Read the model definition and answer for the solid it produces. Units are mm, in the model's axes. A direction names the side the tool comes from. Round coordinates to 2 decimals unless told otherwise and drop trailing zeros. Loops run counter-clockwise (first coordinate to the right, second up) from the corner with the lowest first, then second, coordinate; pieces in that order, holes last. Notation, with made-up numbers: M -37.5,72 L -5.5,72 A23 ccw -5.5,110 Z; hole C 75,39 d4. An arc over 180 degrees is marked long. Answer as CSV lines item,"result".
```python
from build123d import *

# Parameters (mm, degrees)
SKETCH1_R           = 120.65
SKETCH1_R_2         = 7.5
SKETCH1_R_3         = 4
BOSS_EXTRUDE1_DEPTH = 2
SKETCH2_R           = 11.5
SKETCH2_R_2         = 7.5
BOSS_EXTRUDE2_DEPTH = 60
BOSS_EXTRUDE3_DEPTH = 2
CHAMFER1_SIZE       = 3
CHAMFER8_SIZE       = 2


with BuildPart() as part:
    # Sketch1 → Boss-Extrude1 (new body)
    with BuildSketch(Plane(origin=(0, 0, 0), x_dir=(1, 0, 0), z_dir=(0, 1, 0))):
        with Locations(Location((0, 0, 0), (0, 0, 270))):
            Circle(SKETCH1_R)
        with Locations(Location((0, 0, 0), (0, 0, 270))):
            Circle(SKETCH1_R_2, mode=Mode.SUBTRACT)
        with Locations(Location((-85, 0, 0), (0, 0, 270))):
            Circle(SKETCH1_R_3, mode=Mode.SUBTRACT)
        with Locations(Location((-42.5, 73.612159322, 0), (0, 0, 270))):
            Circle(SKETCH1_R_3, mode=Mode.SUBTRACT)
        with Locations(Location((42.5, 73.612159322, 0), (0, 0, 270))):
            Circle(SKETCH1_R_3, mode=Mode.SUBTRACT)
        with Locations(Location((85, 0, 0), (0, 0, 270))):
            Circle(SKETCH1_R_3, mode=Mode.SUBTRACT)
        with Locations(Location((42.5, -73.612159322, 0), (0, 0, 270))):
            Circle(SKETCH1_R_3, mode=Mode.SUBTRACT)
        with Locations(Location((-42.5, -73.612159322, 0), (0, 0, 270))):
            Circle(SKETCH1_R_3, mode=Mode.SUBTRACT)
        with Locations(Location((-110, 0, 0), (0, 0, 270))):
            Circle(SKETCH1_R_3, mode=Mode.SUBTRACT)
        with Locations(Location((-55, 95.262794416, 0), (0, 0, 270))):
            Circle(SKETCH1_R_3, mode=Mode.SUBTRACT)
        with Locations(Location((55, 95.262794416, 0), (0, 0, 270))):
            Circle(SKETCH1_R_3, mode=Mode.SUBTRACT)
        with Locations(Location((110, 0, 0), (0, 0, 270))):
            Circle(SKETCH1_R_3, mode=Mode.SUBTRACT)
        with Locations(Location((55, -95.262794416, 0), (0, 0, 270))):
            Circle(SKETCH1_R_3, mode=Mode.SUBTRACT)
        with Locations(Location((-55, -95.262794416, 0), (0, 0, 270))):
            Circle(SKETCH1_R_3, mode=Mode.SUBTRACT)
        with Locations(Location((-11.320321377, 99.357185568, 0), (0, 0, 270))):
            Circle(SKETCH1_R_3, mode=Mode.SUBTRACT)
        with Locations(Location((11.320321377, 99.357185568, 0), (0, 0, 270))):
            Circle(SKETCH1_R_3, mode=Mode.SUBTRACT)
        with Locations(Location((91.706007439, 39.874906893, 0), (0, 0, 270))):
            Circle(SKETCH1_R_3, mode=Mode.SUBTRACT)
        with Locations(Location((80.385686062, 59.482278675, 0), (0, 0, 270))):
            Circle(SKETCH1_R_3, mode=Mode.SUBTRACT)
        with Locations(Location((80.385686062, -59.482278675, 0), (0, 0, 270))):
            Circle(SKETCH1_R_3, mode=Mode.SUBTRACT)
        with Locations(Location((91.706007439, -39.874906893, 0), (0, 0, 270))):
            Circle(SKETCH1_R_3, mode=Mode.SUBTRACT)
        with Locations(Location((-11.320321377, -99.357185568, 0), (0, 0, 270))):
            Circle(SKETCH1_R_3, mode=Mode.SUBTRACT)
        with Locations(Location((11.320321377, -99.357185568, 0), (0, 0, 270))):
            Circle(SKETCH1_R_3, mode=Mode.SUBTRACT)
        with Locations(Location((-91.706007439, -39.874906893, 0), (0, 0, 270))):
            Circle(SKETCH1_R_3, mode=Mode.SUBTRACT)
        with Locations(Location((-80.385686062, -59.482278675, 0), (0, 0, 270))):
            Circle(SKETCH1_R_3, mode=Mode.SUBTRACT)
        with Locations(Location((-80.385686062, 59.482278675, 0), (0, 0, 270))):
            Circle(SKETCH1_R_3, mode=Mode.SUBTRACT)
        with Locations(Location((-91.706007439, 39.874906893, 0), (0, 0, 270))):
            Circle(SKETCH1_R_3, mode=Mode.SUBTRACT)
    extrude(amount=BOSS_EXTRUDE1_DEPTH)

    # Sketch2 → Boss-Extrude2 (add)
    with BuildSketch(Plane(origin=(0, 2, 0), x_dir=(1, 0, 0), z_dir=(0, 1, 0))):
        with Locations(Location((0, 0, 0), (0, 0, 270))):
            Circle(SKETCH2_R)
        with Locations(Location((0, 0, 0), (0, 0, 270))):
            Circle(SKETCH2_R_2, mode=Mode.SUBTRACT)
    extrude(amount=BOSS_EXTRUDE2_DEPTH)

    # Sketch3 → Revolve1 (revolve)
    with BuildSketch(Plane.XY, mode=Mode.PRIVATE) as revolve1_sk:
        with BuildLine():
            Line((0, 0), (15, 0))
            ThreePointArc((15, 0), (14.880445444, -1.890064387), (14.523687548, -3.75))
            ThreePointArc((14.523687548, -3.75), (12.744320544, -6.452847075), (9.682458366, -7.5))
            Line((9.682458366, -7.5), (0, -7.5))
            Line((0, -7.5), (0, 0))
        make_face()
    revolve(revolve1_sk.sketch.rotate(Axis((0, 0, 0), (0, -1, 0)), 90), axis=Axis((0, 0, 0), (0, -1, 0)))

    # Sketch4 → Boss-Extrude3 (add)
    with BuildSketch(Plane.XZ):
        with BuildLine():
            Line((-19, 90), (19, 90))
            Line((19, 90), (19, 105))
            Line((19, 105), (0.479917223, 168.358177922))
            ThreePointArc((0.479917223, 168.358177922), (0, 168.717894426), (-0.479917223, 168.358177922))
            Line((-0.479917223, 168.358177922), (-19, 105))
            Line((-19, 105), (-19, 90))
        make_face()
        with BuildLine():
            Line((81.432667397, -68.954482672), (145.562500404, -84.594709468))
            ThreePointArc((145.562500404, -84.594709468), (146.113982646, -84.358947213), (146.042417627, -83.763468454))
            Line((146.042417627, -83.763468454), (100.432667397, -36.045517328))
            Line((100.432667397, -36.045517328), (87.442286341, -28.545517328))
            Line((87.442286341, -28.545517328), (68.442286341, -61.454482672))
            Line((68.442286341, -61.454482672), (81.432667397, -68.954482672))
        make_face()
        with BuildLine():
            Line((-100.432667397, -36.045517328), (-146.042417627, -83.763468454))
            ThreePointArc((-146.042417627, -83.763468454), (-146.113982646, -84.358947213), (-145.562500404, -84.594709468))
            Line((-145.562500404, -84.594709468), (-81.432667397, -68.954482672))
            Line((-81.432667397, -68.954482672), (-68.442286341, -61.454482672))
            Line((-68.442286341, -61.454482672), (-87.442286341, -28.545517328))
            Line((-87.442286341, -28.545517328), (-100.432667397, -36.045517328))
        make_face()
    extrude(amount=BOSS_EXTRUDE3_DEPTH)

    # Chamfer1
    chamfer1_edges = [part.edges().sort_by_distance(p)[0] for p in [
        (0, 2, -11.5),
    ]]
    chamfer(chamfer1_edges, length=CHAMFER1_SIZE)

    # Chamfer8
    # the kernel refuses this chamfer: 2 mm, written as the material it takes off along each edge
    with BuildSketch(Plane(origin=(-94.391126841, -2, -29.724721105), x_dir=(0, 1, 0), z_dir=(-0.690957517475874, 0, -0.7228953652110223)), Plane(origin=(-150.55940651, -2, -85.813373872), x_dir=(0, 1, 0), z_dir=(0.9715245092887052, 0, 0.2369390804644533)), Plane(origin=(0.963141497, -2, 173.294957752), x_dir=(0, 1, 0), z_dir=(-0.2805669918128247, 0, -0.9598344456754521)), Plane(origin=(21.453199823, -2, 96.607474288), x_dir=(0, 1, 0), z_dir=(-0.2805669918128244, 0, 0.9598344456754522)), Plane(origin=(149.596265013, -2, -87.48158388), x_dir=(0, 1, 0), z_dir=(-0.6909575174758892, 0, 0.7228953652110078)), Plane(origin=(72.937927017, -2, -66.882753184), x_dir=(0, 1, 0), z_dir=(0.9715245092887104, 0, -0.23693908046443202))) as chamfer8_piece_1:
        Polygon((CHAMFER8_SIZE, 0), (0, CHAMFER8_SIZE), (0, 0), align=None)
    extrude(amount=79.896573633, mode=Mode.SUBTRACT)
    with BuildSketch(Plane(origin=(145.680969944, -2, -84.108947213), x_dir=(-0.2369390804643702, 0, -0.9715245092887255), z_dir=(-0.9715245092887255, 0, 0.2369390804643702))) as chamfer8_piece_2_section:
        Polygon((0.5, -CHAMFER8_SIZE), (0, -1.5), (0, 0), (0.5, 0), align=None)
    chamfer8_piece_2 = revolve(axis=Axis((145.680969944, -2, -84.108947213), (0, -1, 0)), revolution_arc=147.411905087, mode=Mode.PRIVATE)
    chamfer8_piece_2 = split(chamfer8_piece_2, bisect_by=Plane(origin=(145.858674254, -1.25, -83.380303831), z_dir=(-0.16754123052450473, -0.7071067811865483, -0.6869715686069793)), keep=Keep.TOP, mode=Mode.PRIVATE)
    add(chamfer8_piece_2, mode=Mode.SUBTRACT)
    with BuildSketch(Plane(origin=(145.680969944, -2, -84.108947213), x_dir=(-0.2369390804643702, 0, -0.9715245092887255), z_dir=(-0.9715245092887255, 0, 0.2369390804643702))) as chamfer8_piece_3_section:
        Polygon((0.5, -CHAMFER8_SIZE), (0, -1.5), (0, 0), (0.5, 0), align=None)
    chamfer8_piece_3 = revolve(axis=Axis((145.680969944, -2, -84.108947213), (0, -1, 0)), revolution_arc=147.411905087, mode=Mode.PRIVATE)
    chamfer8_piece_3 = split(chamfer8_piece_3, bisect_by=Plane(origin=(145.13879842, -1.25, -84.627165351), z_dir=(0.5111642148290308, -0.7071067811865457, 0.4885807461190251)), keep=Keep.TOP, mode=Mode.PRIVATE)
    add(chamfer8_piece_3, mode=Mode.SUBTRACT)
    with BuildSketch(Plane(origin=(0, -2, 168.217894426), x_dir=(0.9598344456754415, 0, 0.2805669918128611), z_dir=(0.2805669918128611, 0, -0.9598344456754415))) as chamfer8_piece_4_section:
        Polygon((0.5, -CHAMFER8_SIZE), (0, -1.5), (0, 0), (0.5, 0), align=None)
    chamfer8_piece_4 = revolve(axis=Axis((0, -2, 168.217894426), (0, -1, 0)), revolution_arc=147.411905087, mode=Mode.PRIVATE)
    chamfer8_piece_4 = split(chamfer8_piece_4, bisect_by=Plane(origin=(-0.719875834, -1.25, 168.007469182), z_dir=(0.678705445353544, -0.7071067811865469, 0.19839082248795895)), keep=Keep.TOP, mode=Mode.PRIVATE)
    add(chamfer8_piece_4, mode=Mode.SUBTRACT)
    with BuildSketch(Plane(origin=(0, -2, 168.217894426), x_dir=(0.9598344456754415, 0, 0.2805669918128611), z_dir=(0.2805669918128611, 0, -0.9598344456754415))) as chamfer8_piece_5_section:
        Polygon((0.5, -CHAMFER8_SIZE), (0, -1.5), (0, 0), (0.5, 0), align=None)
    chamfer8_piece_5 = revolve(axis=Axis((0, -2, 168.217894426), (0, -1, 0)), revolution_arc=147.411905087, mode=Mode.PRIVATE)
    chamfer8_piece_5 = split(chamfer8_piece_5, bisect_by=Plane(origin=(0.719875834, -1.25, 168.007469182), z_dir=(-0.6787054453535436, -0.707106781186547, 0.19839082248795903)), keep=Keep.TOP, mode=Mode.PRIVATE)
    add(chamfer8_piece_5, mode=Mode.SUBTRACT)
    with BuildSketch(Plane(origin=(-145.680969944, -2, -84.108947213), x_dir=(-0.7228953652110097, 0, 0.6909575174758872), z_dir=(0.6909575174758872, 0, 0.7228953652110097))) as chamfer8_piece_6_section:
        Polygon((0.5, -CHAMFER8_SIZE), (0, -1.5), (0, 0), (0.5, 0), align=None)
    chamfer8_piece_6 = revolve(axis=Axis((-145.680969944, -2, -84.108947213), (0, -1, 0)), revolution_arc=147.411905087, mode=Mode.PRIVATE)
    chamfer8_piece_6 = split(chamfer8_piece_6, bisect_by=Plane(origin=(-145.13879842, -1.25, -84.627165351), z_dir=(-0.5111642148290398, -0.7071067811865479, 0.488580746119013)), keep=Keep.TOP, mode=Mode.PRIVATE)
    add(chamfer8_piece_6, mode=Mode.SUBTRACT)
    with BuildSketch(Plane(origin=(-145.680969944, -2, -84.108947213), x_dir=(-0.7228953652110097, 0, 0.6909575174758872), z_dir=(0.6909575174758872, 0, 0.7228953652110097))) as chamfer8_piece_7_section:
        Polygon((0.5, -CHAMFER8_SIZE), (0, -1.5), (0, 0), (0.5, 0), align=None)
    chamfer8_piece_7 = revolve(axis=Axis((-145.680969944, -2, -84.108947213), (0, -1, 0)), revolution_arc=147.411905087, mode=Mode.PRIVATE)
    chamfer8_piece_7 = split(chamfer8_piece_7, bisect_by=Plane(origin=(-145.858674254, -1.25, -83.380303831), z_dir=(0.16754123052451989, -0.7071067811865478, -0.6869715686069761)), keep=Keep.TOP, mode=Mode.PRIVATE)
    add(chamfer8_piece_7, mode=Mode.SUBTRACT)


solid = part.part
```
1) Find section D-D, the plane z = 136. Give the vertices of the cut face in (x, y), then the cut area to 3 significant figures.
Evaluation:
outline,"M -9.94,0 L -7.85,-2 L 7.85,-2 L 9.94,0 Z"
area,"35.6 mm^2"
2) Each of these flat-tipped pins is pushed along its axis until it touches: P1, Ø10.5, axis at x = -85, z = 0, coming from the -Y side; P2, Ø1.5, axis at x = 38.5, z = -8, coming from the +Y side; P3, Ø2, axis at y = -0.5, z = 100.5, coming from the -X side. Where does it stop, or does it pass through?
Evaluation:
P1,"stops at y = 0"
P2,"stops at y = 2"
P3,"stops at x = -68.04"
3) Straight lines are drawn through the part: line 1 (Y direction, x = -47, z = 26); line 2 (X direction, y = 37, z = 2.5). For each, find the intervals that lie inside material, in ascending order.
Evaluation:
line 1,"y = 0 to 2"
line 2,"x = -11.22 to -7.07, 7.07 to 11.22"
4) Find section A-A, the plane x = 55. Give the vertices of the cut face in (y, z), then the cut area to 3 significant figures.
Evaluation:
outline,"M 0,-107.38 L 2,-107.38 L 2,-99.26 L 0,-99.26 Z; M 0,-91.26 L 2,-91.26 L 2,91.26 L 0,91.26 Z; M 0,99.26 L 2,99.26 L 2,107.38 L 0,107.38 Z"
area,"398 mm^2"
5) Find section C-C, the plane y = 57.5. Give the vertices of the cut face in (x, z).
Evaluation:
outline,"C 0,0 d23; hole C 0,0 d15"
6) A tool of negligible diameter and unlimited length cuts with its end or side. For faces 1 (the cylindrical face through (43.7, 0.99, 77.43)), 2 (the flat face through (-92, 0, -40)), from which of +Z, -Z, +X, -X, +Y, -Y can it reach the whole face along a straight path? Write none if from no direction.
Evaluation:
face 1,"+Y, -Y"
face 2,"+Y"
7) Find section B-B, the plane z = 0. Count the separate pieces of the cut face and the enclosed holes in it, then the cut area to 3 significant figures.
Evaluation:
separate pieces,"5"
enclosed holes,"0"
area,"1,090 mm^2"
8) Determine the mould class of faces 3 (the conical face through (3.5, 4.85, 11.11)), 4 (the flat face through (92.585, -0.986, -31.515)), 5 (the flat face through (78.075, -0.986, -44.77)) for opening direction X: released by +X, released by -X, zero draft, split by the parting line, or undercut.
Evaluation:
face 3,"split by the parting line"
face 4,"released by +X"
face 5,"undercut"
